```python
from build123d import *

# Parameters (mm, degrees)
F1_DEPTH = 63.5
F2_DEPTH = 25.4
F3_DEPTH = 7.9375
F0_W     = 25.4
F0_H     = 19.05
F4_DEPTH = 25.4
F6_R     = 6.35


with BuildPart() as f1:
    # F0 (on Front) → F1 (new body, symmetric)
    with BuildSketch(Plane.XZ):
        Polygon((22.225, 9.525), (-41.275, 9.525), (-41.275, -9.525), (41.275, -9.525), (41.275, 9.525), align=None)
    extrude(amount=F1_DEPTH, both=True)

    # F0 (on Front) → F2 (join, symmetric)
    with BuildSketch(Plane.XZ):
        with BuildLine():
            Line((22.225, 27.1335136465), (22.225, 9.525))
            Line((22.225, 9.525), (41.275, 9.525))
            Line((41.275, 9.525), (41.275, 27.1335136465))
            ThreePointArc((41.275, 27.1335136465), (46.6756561073, 39.0626269839), (59.2030308685, 42.8752))
            Line((59.2030308685, 42.8752), (60.325, 42.8752))
            Line((60.325, 42.8752), (60.325, 61.9252))
            Line((60.325, 61.9252), (60.1986366915, 61.9252))
            add(Edge.make_bspline(
                [(55.5778495322, 62.02311049), (57.0926075375, 62.0086737376), (58.6326298587, 61.9761317105), (60.1986366915, 61.9252)],
                knots=[111.0214759669, 111.0214759669, 111.0214759669, 111.0214759669, 114.2045529016, 114.2045529016, 114.2045529016, 114.2045529016], degree=3))
            ThreePointArc((55.5778495322, 62.02311049), (31.904574869, 51.2669786889), (22.225, 27.1335136465))
        make_face()
    extrude(amount=F2_DEPTH, both=True)

    # F0 (on Front) → F3 (join, symmetric)
    with BuildSketch(Plane.XZ):
        with BuildLine():
            add(Edge.make_bspline(
                [(-41.275, 9.525), (-19.3530475972, 41.0047273115), (2.745111609, 62.5266451514), (55.5778495322, 62.02311049)],
                knots=[0, 0, 0, 0, 111.0214759669, 111.0214759669, 111.0214759669, 111.0214759669], degree=3))
            Line((-41.275, 9.525), (22.225, 9.525))
            Line((22.225, 9.525), (22.225, 27.1335136465))
            ThreePointArc((22.225, 27.1335136465), (31.904574869, 51.2669786889), (55.5778495322, 62.02311049))
        make_face()
    extrude(amount=F3_DEPTH, both=True)

    # F0 (on Front) → F4 (join, symmetric)
    with BuildSketch(Plane.XZ):
        with Locations((73.025, 52.4002)):
            Rectangle(F0_W, F0_H)
    extrude(amount=F4_DEPTH, both=True)

    # F0 (on Front) → F5 (revolve)
    with BuildSketch(Plane.XZ):
        Polygon((85.725, 66.675), (85.725, 61.9252), (85.725, 42.8752), (85.725, 38.1), (111.125, 38.1), (111.125, 66.675), align=None)
    revolve(axis=Axis((85.725, 0, 52.3875), (0, 0, 1)))

    # F6
    f6_edges = [f1.edges().sort_by_distance(p)[0] for p in [
        (-41.275, -63.5, 0),
        (41.275, -63.5, 0),
        (-41.275, 63.5, 0),
        (41.275, 63.5, 0),
    ]]
    fillet(f6_edges, radius=F6_R)


solid = f1.part
```
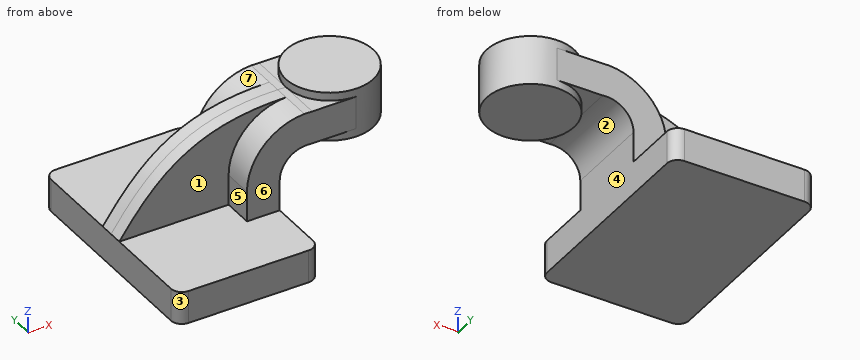
CAD build for the part. Positions are in the model's coordinates, mm. Face numbers are marked on the shaded views. A direction names the side the tool comes from. Round coordinates to 2 decimals unless told otherwise and drop trailing zeros. Write each loop counter-clockwise with the first axis right and the second up, starting at its lowest first coordinate (ties: lowest second). Pieces come first, ordered by that corner, then holes. Notation, with made-up numbers: (81.25, -34.5) - (95.25, -34.5) arc R11 ccw to (95.25, -26.5) - close; hole circle Ø8 at (49.25, 86). An arc over 180 degrees is marked (long way). Return JSON: item names as keys, results as strings. Group by question number.
Item 1: Band-saw the part on B-B on x = 79.5. List the corners of the cut face in (y, z) (3 decimals).
Item 2: Probe probe 1 along Z at (x, y) = (30, 57) (3 decimals); probe 2 along X at (y, z) = (-23, 40); probe 3 along X at (y, z) = (6.5, 41.5). List the from-to ranges inside material, lowest first.
Item 3: 3-axis set-ups, long thin cutter, end or side, ignore diameter. For the marked faces 5, 6 and 7: which of +Z, -Z, +X, -X, +Y, -Y reach the whole face in a straight line?
Item 4: Band-saw the part on D-D on x = 97. List the corners of the cut face in (y, z) (3 decimals).
Item 5: Band-saw the part on A-A on z = 7.5. List the corners of the cut face in (x, y) (3 decimals), plus the area to 3 significant figures.
Item 6: Mould opens along X. For the marked faces 1, 2, 3 and 4 say: +X half, -X half, draft (parallel to the pull), parting line (faces both ways), or undercut.
Item 7: Flat gauge pins, fed straight in: pin 1 Ø16.5 at (x, y) = (-16, -22.5) entering from +Z (3 decimals); pin 2 Ø6 at (x, z) = (12.5, 56) entering from -Y; pin 3 Ø10 at (x, z) = (5.5, 27.5) entering from +Y; pin 4 Ø3 at (x, z) = (44.5, 15.5) entering from -Y. Where does each tip first touch, or does it go through?
Item 8: Band-saw the part on C-C on y = 45. List the corners of the cut face in (x, z) (3 decimals), plus the area to 3 significant figures.
Resolved:
{
 "1": {"outline": "(-25.4, 42.875) - (-24.625, 42.875) - (-24.625, 38.1) - (24.625, 38.1) - (24.625, 42.875) - (25.4, 42.875) - (25.4, 61.925) - (24.625, 61.925) - (24.625, 66.675) - (-24.625, 66.675) - (-24.625, 61.925) - (-25.4, 61.925) - close"},
 "2": {"probe 1": "z = -9.525 to 9.525", "probe 2": "x = 24.68 to 47.85, 74.95 to 96.5", "probe 3": "x = -13.24 to 50.4, 61.17 to 110.28"},
 "3": {"face 5": "+Z, -X, -Y", "face 6": "+Z, +X, -X, -Y", "face 7": "+Z, -X, +Y"},
 "4": {"outline": "(-22.76, 38.1) - (22.76, 38.1) - (22.76, 66.675) - (-22.76, 66.675) - close"},
 "5": {"outline": "(-41.275, -57.15) arc R6.35 ccw to (-34.925, -63.5) - (34.925, -63.5) arc R6.35 ccw to (41.275, -57.15) - (41.275, 57.15) arc R6.35 ccw to (34.925, 63.5) - (-34.925, 63.5) arc R6.35 ccw to (-41.275, 57.15) - close", "area": "10,400 mm²"},
 "6": {"face 1": "draft", "face 2": "undercut", "face 3": "-X half", "face 4": "+X half"},
 "7": {"pin 1": "stops at z = 9.525", "pin 2": "stops at y = -7.94", "pin 3": "stops at y = 7.94", "pin 4": "passes through"},
 "8": {"outline": "(-41.275, -9.525) - (41.275, -9.525) - (41.275, 9.525) - (-41.275, 9.525) - close", "area": "1,570 mm²"}
}
